Source: three-view drawing plus pictorial views. Frame: mm from the lowest corner of the part. A direction names the side the tool comes from. Round coordinates to 2 decimals unless told otherwise and drop trailing zeros. Loops run counter-clockwise (first coordinate to the right, second up) from the corner with the lowest first, then second, coordinate; pieces in that order, holes last. Notation, with made-up numbers: M -28,-21 L 5,-21 A29 cw 5,2 Z; hole C 71,87.25 d10. An arc over 180 degrees is marked long. Answer as a JSON object with one key per item and string values.
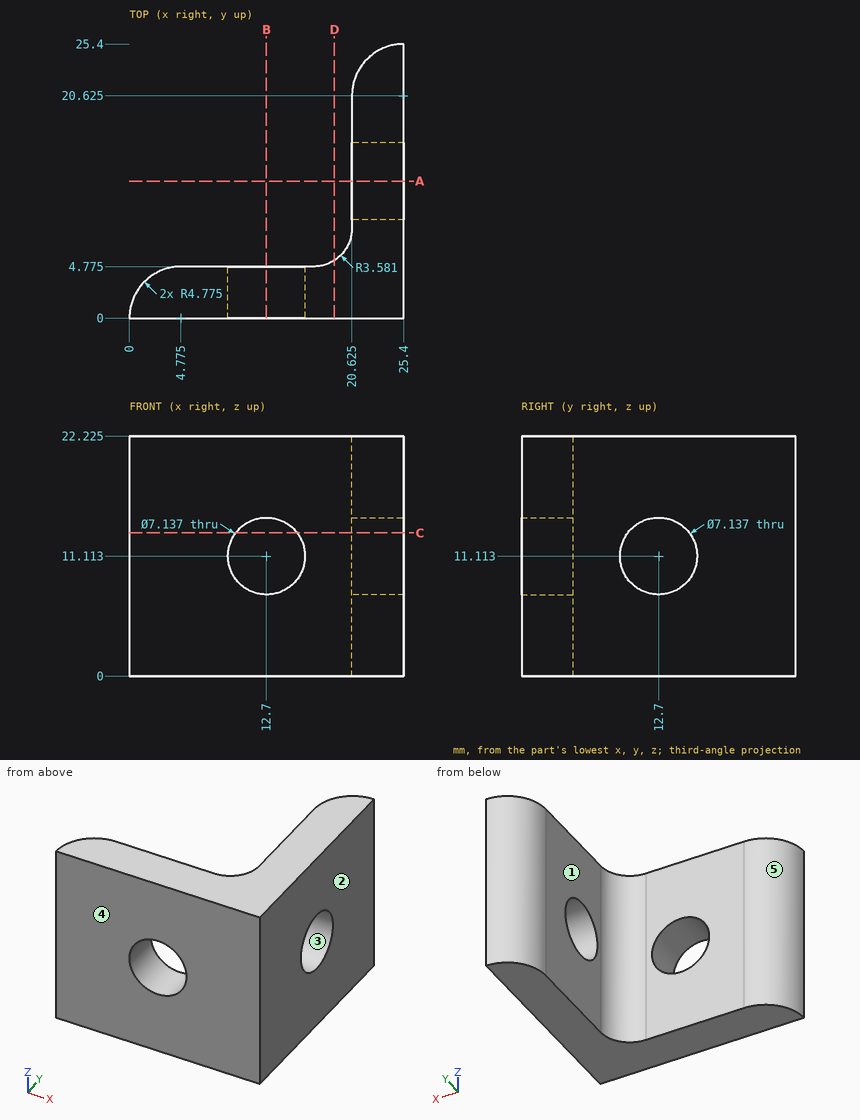
1) First-contact query: pin 1 (12 mm diameter, centred on y = 13, z = 10, fed in from -X); pin 2 (6 mm diameter, centred on y = 13.5, z = 12.5, fed in from -X) (1 decimal); pin 3 (6.5 mm diameter, centred on y = 12.7, z = 11.11, fed in from -X); pin 4 (10 mm diameter, centred on x = 11.5, z = 7.5, fed in from +Y) (1 decimal). Flat tips, straight axial feed; report the tip coordinate or a pass-through.
Geometry results:
{"pin 1": "x = 20.36", "pin 2": "x = 20.6", "pin 3": "through", "pin 4": "y = 4.8"}
2) Cut plane A-A on y = 12.7. Return the cut outline in (x, z) (1 decimal).
Geometry results:
{"outline": "M 20.6,0 L 25.4,0 L 25.4,7.5 L 20.6,7.5 Z; M 20.6,14.7 L 25.4,14.7 L 25.4,22.2 L 20.6,22.2 Z"}
3) Cut plane D-D on x = 19. Return the cut outline in (y, z) (1 decimal).
Geometry results:
{"outline": "M 0,0 L 5.4,0 L 5.4,22.2 L 0,22.2 Z"}
4) Cut plane C-C on z = 13.25. Count the separate pieces of the cut face and the enclosed holes in it, and give its area (3 significant figures).
Geometry results:
{"separate pieces": "3", "enclosed holes": "0", "area": "158 mm2"}
5) Set-up query: the marked faces 1 and 2. Return all of +Z, -Z, +X, -X, +Y, -Y with unobstructed straight access to the full face (end or side cutting, diameter ignored); none if empty.
Geometry results:
{"face 1": "+Z, -Z, -X, +Y", "face 2": "+Z, -Z, +X, +Y, -Y"}
6) Line query: probe 1 along Z at (x, y) = (12.7, 1) (1 decimal); probe 2 along X at (y, z) = (9.75, 14.5) (1 decimal); probe 3 along Y at (x, z) = (5.75, 4.75) (1 decimal). Output: solid intervals per line, ascending.
Geometry results:
{"probe 1": "0 to 7.5, 14.7 to 22.2", "probe 2": "20.6 to 25.4", "probe 3": "0 to 4.8"}
7) Pull-direction query (Y, two-part tool) for the marked faces 3, 4 and 5; classes: +Y half, -Y half, draft (parallel to the pull), parting line (faces both ways), or undercut.
Geometry results:
{"face 3": "undercut", "face 4": "-Y half", "face 5": "+Y half"}
8) Cut plane B-B on x = 12.7. Return the cut outline in (y, z) (1 decimal).
Geometry results:
{"outline": "M 0,0 L 4.8,0 L 4.8,7.5 L 0,7.5 Z; M 0,14.7 L 4.8,14.7 L 4.8,22.2 L 0,22.2 Z"}
